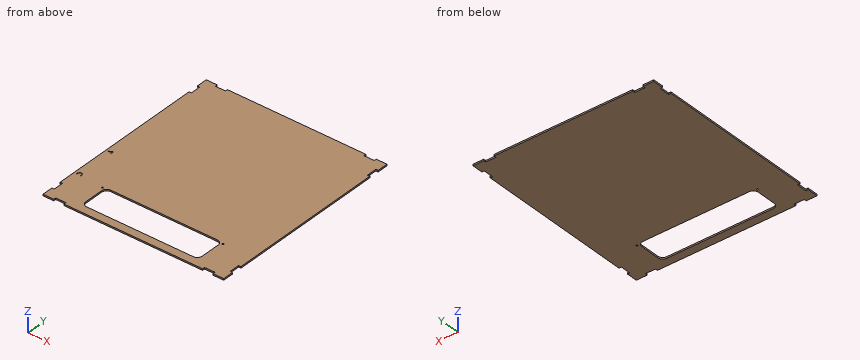
```python
from build123d import *

# Parameters (mm, degrees)
SKETCH_R     = 1.5
PAD_DEPTH    = 3
POCKET_DEPTH = 1


with BuildPart() as part:
    # Sketch → Pad (new body)
    with BuildSketch(Plane.XY):
        Polygon((-173.9, 176.1), (-178.5, 176.1), (-178.5, 197.5), (-157.1, 197.5), (-157.1, 192.9), (-136.9, 192.9), (-136.9, 197.5), (136.9, 197.5), (136.9, 192.9), (157.1, 192.9), (157.1, 197.5), (178.5, 197.5), (178.5, 176.1), (173.9, 176.1), (173.9, 155.9), (178.5, 155.9), (178.5, -155.9), (173.9, -155.9), (173.9, -176.1), (178.5, -176.1), (178.5, -197.5), (157.1, -197.5), (157.1, -192.9), (136.9, -192.9), (136.9, -197.5), (-136.9, -197.5), (-136.9, -192.9), (-157.1, -192.9), (-157.1, -197.5), (-178.5, -197.5), (-178.5, -176.1), (-173.9, -176.1), (-173.9, -155.9), (-178.5, -155.9), (-178.5, 155.9), (-173.9, 155.9), align=None)
        with Locations((-119, -126.3)):
            Circle(SKETCH_R, mode=Mode.SUBTRACT)
        with Locations((119, -126.3)):
            Circle(SKETCH_R, mode=Mode.SUBTRACT)
        with BuildLine():
            Line((-105, -123.5), (105, -123.5))
            ThreePointArc((115, -133.5), (112.071068, -126.428932), (105, -123.5))
            Line((115, -133.5), (115, -171.5))
            ThreePointArc((105, -181.5), (112.071068, -178.571068), (115, -171.5))
            Line((105, -181.5), (-105, -181.5))
            ThreePointArc((-115, -171.5), (-112.071068, -178.571068), (-105, -181.5))
            Line((-115, -171.5), (-115, -133.5))
            ThreePointArc((-105, -123.5), (-112.071068, -126.428932), (-115, -133.5))
        make_face(mode=Mode.SUBTRACT)
    extrude(amount=PAD_DEPTH)

    # Sketch001 (on Face48 of Pad) → Pocket (cut)
    with BuildSketch(Plane.XY.offset(3)):
        with BuildLine():
            Line((-170.9, -45.75), (-173.9, -45.75))
            Line((-173.9, -45.75), (-173.9, -44.25))
            Line((-173.9, -44.25), (-170.9, -44.25))
            ThreePointArc((-168.650001, -42.00001), (-170.240987, -42.659016), (-170.9, -44.25))
            Line((-168.650001, -42.00001), (-167.150001, -42.00001))
            Line((-167.150001, -42.00001), (-167.150001, -43.12501))
            Line((-167.150001, -43.12501), (-165.650001, -43.12501))
            Line((-165.650001, -43.12501), (-165.650001, -43.87501))
            Line((-165.650001, -43.87501), (-167.150001, -43.87501))
            Line((-167.150001, -43.87501), (-167.150001, -46.12501))
            Line((-167.150001, -46.12501), (-165.650001, -46.12501))
            Line((-165.650001, -46.12501), (-165.650001, -46.87501))
            Line((-165.650001, -46.87501), (-167.150001, -46.87501))
            Line((-167.150001, -46.87501), (-167.150001, -48.00001))
            Line((-167.150001, -48.00001), (-168.650001, -48.00001))
            ThreePointArc((-170.9, -45.75), (-170.240994, -47.340997), (-168.650001, -48.00001))
        make_face()
        with BuildLine():
            ThreePointArc((-165.65, -120), (-168.65, -117), (-171.65, -120))
            Line((-171.65, -120), (-171.65, -123))
            Line((-171.65, -123), (-172.4, -123))
            ThreePointArc((-172.4, -120), (-173.9, -121.5), (-172.4, -123))
            ThreePointArc((-164.9, -120), (-168.65, -116.25), (-172.4, -120))
            ThreePointArc((-164.9, -123), (-163.4, -121.5), (-164.9, -120))
            Line((-165.65, -123), (-164.9, -123))
            Line((-165.65, -120), (-165.65, -123))
        make_face()
    extrude(amount=-POCKET_DEPTH, mode=Mode.SUBTRACT)


solid = part.part
```
Can you work these out from the model? Positions are in its coordinate system, mm. Give positions to 0.01 mm unless a question says otherwise; leave off trailing zeros. Write each loop counter-clockwise with the first axis right and the second up, starting at its lowest first coordinate (ties: lowest second). Pieces come first, ordered by that corner, then holes. Notation, with made-up numbers: (46.5, 86) - (54.5, 86) arc R14 cw to (54.5, 111) - close; hole circle Ø2 at (49.25, 79.5). An arc over 180 degrees is marked (long way). Write item = value, one per line. Start each with the question number.
1. Please list where these lines run through material, in increasing order: line 1 (Y direction, x = 56, z = 2.05); line 2 (Y direction, x = -119, z = 1); line 3 (X direction, y = -150.5, z = 1.8).
2. Imagine slicing it at B-B (y = -142). Please give me the cut outline in (x, z), and give its area (3 significant figures).
3. Imagine slicing it at A-A (x = 34.5). Please give me the cut outline in (y, z).
Worked answers:
q1.line_1 = -197.5 to -181.5, -123.5 to 197.5
q1.line_2 = -197.5 to -127.8, -124.8 to 197.5
q1.line_3 = -178.5 to -115, 115 to 178.5
q2.outline = (-178.5, 0) - (-115, 0) - (-115, 3) - (-178.5, 3) - close; (115, 0) - (178.5, 0) - (178.5, 3) - (115, 3) - close
q2.area = 381 mm2
q3.outline = (-197.5, 0) - (-181.5, 0) - (-181.5, 3) - (-197.5, 3) - close; (-123.5, 0) - (197.5, 0) - (197.5, 3) - (-123.5, 3) - close
